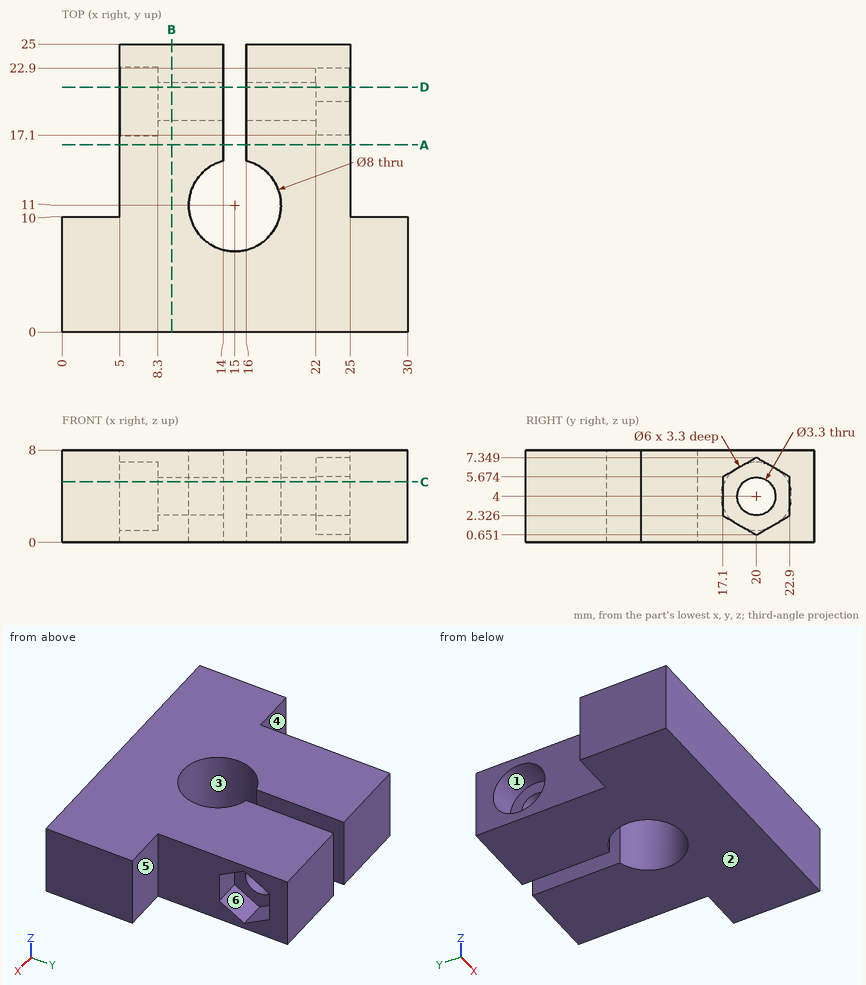
The figure shows three views and two pictorial views of one solid part (mm, origin at its lowest corner). Answer the questions. A direction names the side the tool comes from. Give positions to 0.01 mm unless a question says otherwise; leave off trailing zeros. Order: outer loops, then holes, each group sorted by start corner. A loop starts at its lowest first (then second) coordinate and runs counter-clockwise, first axis right, second up. Notation, with made-up numbers: (41.25, 64.5) -> (92.25, 64.5) arc R11 ccw to (92.25, 70.5) -> close; hole circle Ø11 at (27.25, 19). An arc over 180 degrees is marked (long way). One line per item, written item: value.
1) Determine the mould class of the marked faces 1, 2 and 3 for opening direction Z: pulls with the +Z half, pulls with the -Z half, needs draft (parallel to the pull), parting line crosses it, or undercut.
Reported:
face 1: undercut
face 2: pulls with the -Z half
face 3: needs draft
2) Find section B-B, the plane x = 9.5. Determine the outline of the cut face in (y, z).
Reported:
outline: (0, 0) -> (25, 0) -> (25, 8) -> (0, 8) -> close; hole circle Ø3.3 at (20, 4)
3) A tool of negligible diameter and unlimited length cuts with its end or side. For the marked faces 4, 5 and 6, from which of +Z, -Z, +X, -X, +Y, -Y can it reach the whole face along a straight path? Write none if from no direction.
Reported:
face 4: +Z, -Z, -X, +Y
face 5: +Z, -Z, +X, +Y
face 6: +X
4) Find the intervals of material crossed by line 1 (Y direction, x = 19.45, z = 4); line 2 (X direction, y = 24.25, z = 5.75); line 3 (X direction, y = 19.25, z = 6.25), in increasing order.
Reported:
line 1: y = 0 to 18.35, 21.65 to 25
line 2: x = 5 to 14, 16 to 25
line 3: x = 8.3 to 14, 16 to 22
5) Flat-ended cylindrical pins translate along their axes: P1, Ø3, axis at y = 19, z = 3, coming from the +X side; P2, Ø5, axis at x = 3.5, y = 19.5, coming from the -Z side; P3, Ø1.8, axis at y = 20, z = 4.5, coming from the -X side; P4, Ø2, axis at y = 22, z = 2.5, coming from the +X side. Find the tip coordinate at first contact, or state that the pin passes through.
Reported:
P1: stops at x = 22
P2: stops at z = 0
P3: passes through
P4: stops at x = 25
6) Find section A-A, the plane y = 16.25. Determine the outline of the cut face in (x, z), plus the area to 3 significant figures.
Reported:
outline: (5, 0) -> (14, 0) -> (14, 8) -> (5, 8) -> close; (16, 0) -> (25, 0) -> (25, 8) -> (16, 8) -> close
area: 144 mm^2
7) Find section C-C, the plane z = 5.25. Determine the outline of the cut face in (x, y).
Reported:
outline: (0, 0) -> (30, 0) -> (30, 10) -> (25, 10) -> (25, 17.1) -> (22, 17.1) -> (22, 18.92) -> (16, 18.92) -> (16, 14.87) arc R4 cw (long way) to (14, 14.87) -> (14, 18.92) -> (8.3, 18.92) -> (8.3, 17.27) -> (5, 17.27) -> (5, 10) -> (0, 10) -> close; (5, 22.73) -> (8.3, 22.73) -> (8.3, 21.08) -> (14, 21.08) -> (14, 25) -> (5, 25) -> close; (16, 21.08) -> (22, 21.08) -> (22, 22.9) -> (25, 22.9) -> (25, 25) -> (16, 25) -> close
8) Find section D-D, the plane y = 21.25. Determine the outline of the cut face in (x, z).
Reported:
outline: (5, 0) -> (14, 0) -> (14, 2.92) -> (8.3, 2.92) -> (8.3, 1.27) -> (5, 1.27) -> close; (5, 6.73) -> (8.3, 6.73) -> (8.3, 5.08) -> (14, 5.08) -> (14, 8) -> (5, 8) -> close; (16, 0) -> (25, 0) -> (25, 1.37) -> (22, 1.37) -> (22, 2.92) -> (16, 2.92) -> close; (16, 5.08) -> (22, 5.08) -> (22, 6.63) -> (25, 6.63) -> (25, 8) -> (16, 8) -> close
